Read the model definition and answer for the solid it produces. Units are mm, in the model's axes. Give positions to 0.01 mm unless a question says otherwise; leave off trailing zeros. Return JSON: item names as keys, results as strings.
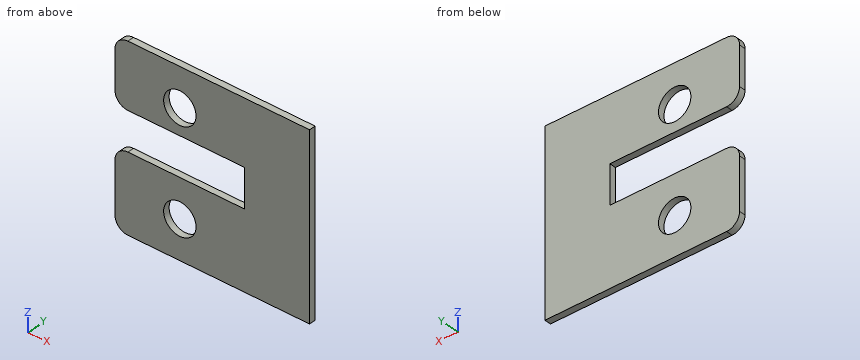
```python
from build123d import *

# Parameters (mm, degrees)
F0_R     = 7.9375
F1_DEPTH = 3.175


# Not quite as in the source:
# - a feature names something its author has since deleted; it is built from what else it names


with BuildPart() as f1:
    # F0 (on Front) → F1 (new body)
    with BuildSketch(Plane.XZ):
        with BuildLine():
            Line((-107.95, 82.55), (-107.95, 63.5))
            ThreePointArc((-107.95, 63.5), (-106.0901280605, 59.0098719395), (-101.6, 57.15))
            Line((-101.6, 57.15), (-44.45, 57.15))
            Line((-44.45, 57.15), (-44.45, 88.9))
            Line((-44.45, 88.9), (-101.6, 88.9))
            ThreePointArc((-101.6, 88.9), (-106.0901280605, 87.0401280605), (-107.95, 82.55))
        make_face()
        with Locations((-76.2, 69.85)):
            Circle(F0_R, mode=Mode.SUBTRACT)
        Polygon((-44.45, 88.9), (-44.45, 57.15), (-44.45, 38.1), (-44.45, 0), (-12.7, 0), (-12.7, 88.9), align=None)
        with BuildLine():
            Line((-44.45, 0), (-44.45, 38.1))
            Line((-44.45, 38.1), (-101.6, 38.1))
            ThreePointArc((-101.6, 38.1), (-106.0901280605, 36.2401280605), (-107.95, 31.75))
            Line((-107.95, 31.75), (-107.95, 6.35))
            ThreePointArc((-107.95, 6.35), (-106.0901280605, 1.8598719395), (-101.6, 0))
            Line((-101.6, 0), (-95.25, 0))
            Line((-95.25, 0), (-44.45, 0))
        make_face()
        with Locations((-76.2, 19.05)):
            Circle(F0_R, mode=Mode.SUBTRACT)
    extrude(amount=F1_DEPTH)


solid = f1.part
```
Q1. Consider L1, parallel to Z at x = -76.2, y = -2.5; L2, parallel to X at y = -3, z = 18.5; L3, parallel to Z at x = -83, y = -1.6. Determine where each line is inside the solid, lowest interval first.
Values:
{"L1": "z = 0 to 11.11, 26.99 to 38.1, 57.15 to 61.91, 77.79 to 88.9", "L2": "x = -107.95 to -84.12, -68.28 to -12.7", "L3": "z = 0 to 14.96, 23.14 to 38.1, 57.15 to 65.76, 73.94 to 88.9"}
Q2. A cutting plane is placed at A-A (x = -76.2). Give the number of separate pieces and of enclosed holes in the cut face, and give its area (3 significant figures).
Values:
{"separate pieces": "4", "enclosed holes": "0", "area": "121 mm²"}
Q3. Given pin 1 (9.5 mm diameter, centred on x = -76.2, z = 69.85, fed in from -Y); pin 2 (20.5 mm diameter, centred on x = -76.2, z = 19.05, fed in from +Y); pin 3 (1.6 mm diameter, centred on y = -1.5, z = 47, fed in from -X), each flat-ended and moving along its own axis, determine where each tip first touches the part or whether it passes through.
Values:
{"pin 1": "passes through", "pin 2": "stops at y = 0", "pin 3": "stops at x = -44.45"}
